Model file for the job. Use its own axes, mm. Give positions to 0.01 mm unless a question says otherwise; leave off trailing zeros. Write each loop counter-clockwise with the first axis right and the second up, starting at its lowest first coordinate (ties: lowest second). Pieces come first, ordered by that corner, then holes. Notation, with made-up numbers: (78.5, -13.75) - (109.5, -13.75) arc R14 cw to (109.5, -8.75) - close; hole circle Ø9 at (27.5, -10.75). An arc over 180 degrees is marked (long way). Use a Markdown table: item, result. Add a question column.
```python
from build123d import *

# Parameters (mm, degrees)
SKETCH_1_W          = 77.1
SKETCH_1_H          = 60
SKETCH_1_R          = 4.1
SKETCH_1_R_2        = 1.6
SKETCH_1_W_2        = 3.1
SKETCH_1_H_2        = 10
EXTRUDE_1_DEPTH     = 3
SKETCH_2_R          = 1.55
SKETCH_2_W          = 21.45
SKETCH_2_H          = 17
CUT_EXTRUDE_1_DEPTH = 49.939784429
SKETCH_3_R          = 4.1
EXTRUDE_2_DEPTH     = 3
FILLET_1_R          = 3


with BuildPart() as part:
    # 草图1 → 凸台-拉伸1 (new body)
    with BuildSketch(Plane.XY):
        Rectangle(SKETCH_1_W, SKETCH_1_H)
        Circle(SKETCH_1_R, mode=Mode.SUBTRACT)
        with Locations((34, 0)):
            Circle(SKETCH_1_R_2, mode=Mode.SUBTRACT)
        with Locations((-34, 0)):
            Circle(SKETCH_1_R_2, mode=Mode.SUBTRACT)
        with Locations((34, -20)):
            Rectangle(SKETCH_1_W_2, SKETCH_1_H_2, mode=Mode.SUBTRACT)
        with Locations((-34, 20)):
            Rectangle(SKETCH_1_W_2, SKETCH_1_H_2, mode=Mode.SUBTRACT)
        with Locations((-34, -20)):
            Rectangle(SKETCH_1_W_2, SKETCH_1_H_2, mode=Mode.SUBTRACT)
        with Locations((34, 20)):
            Rectangle(SKETCH_1_W_2, SKETCH_1_H_2, mode=Mode.SUBTRACT)
    extrude(amount=EXTRUDE_1_DEPTH)

    # 草图2 → 切除-拉伸1 (cut, through all)
    with BuildSketch(Plane.XY.offset(3)):
        with Locations((-34, 25)):
            Circle(SKETCH_2_R)
        with Locations((-34, 15)):
            Circle(SKETCH_2_R)
        with Locations((34, 25)):
            Circle(SKETCH_2_R)
        with Locations((34, 15)):
            Circle(SKETCH_2_R)
        with Locations((34, -15)):
            Circle(SKETCH_2_R)
        with Locations((34, -25)):
            Circle(SKETCH_2_R)
        with Locations((-34, -15)):
            Circle(SKETCH_2_R)
        with Locations((-34, -25)):
            Circle(SKETCH_2_R)
        with Locations((-15.725, 13.5)):
            Rectangle(SKETCH_2_W, SKETCH_2_H)
        with Locations((15.725, 13.5)):
            Rectangle(SKETCH_2_W, SKETCH_2_H)
        with Locations((-15.725, -13.5)):
            Rectangle(SKETCH_2_W, SKETCH_2_H)
        with Locations((15.725, -13.5)):
            Rectangle(SKETCH_2_W, SKETCH_2_H)
    extrude(amount=-CUT_EXTRUDE_1_DEPTH, mode=Mode.SUBTRACT)

    # 草图3 → 凸台-拉伸2 (add)
    # profile 1 of 2: a face of its own
    with BuildSketch(Plane.XY.offset(3)):
        Polygon((-38.55, 30), (-53.55, 12.123696111), (-53.55, -12.123696111), (-38.55, -30), align=None)
        with Locations((-46.5, 0)):
            Circle(SKETCH_3_R, mode=Mode.SUBTRACT)
        with BuildLine():
            Line((-40.55, 19.837873681), (-49.55, 9.112091347))
            Line((-49.55, 9.112091347), (-49.55, 7.503832354))
            ThreePointArc((-49.55, 7.503832354), (-44.736420639, 7.905680732), (-40.55, 5.496135006))
            Line((-40.55, 5.496135006), (-40.55, 19.837873681))
        make_face(mode=Mode.SUBTRACT)
        with BuildLine():
            Line((-49.55, -7.503832354), (-49.55, -9.112091347))
            Line((-49.55, -9.112091347), (-40.55, -19.837873681))
            Line((-40.55, -19.837873681), (-40.55, -5.496135006))
            ThreePointArc((-40.55, -5.496135006), (-44.736420639, -7.905680732), (-49.55, -7.503832354))
        make_face(mode=Mode.SUBTRACT)
    # profile 2 of 2: a face of its own
    with BuildSketch(Plane.XY.offset(3)):
        Polygon((53.55, -12.123696111), (38.55, -30), (38.55, 30), (53.55, 12.123696111), align=None)
        with Locations(Location((46.5, 0, 0), (0, 0, 180))):
            Circle(SKETCH_3_R, mode=Mode.SUBTRACT)
        with BuildLine():
            Line((40.55, -19.837873681), (40.55, -5.496135006))
            ThreePointArc((40.55, -5.496135006), (44.736420639, -7.905680732), (49.55, -7.503832354))
            Line((49.55, -7.503832354), (49.55, -9.112091347))
            Line((49.55, -9.112091347), (40.55, -19.837873681))
        make_face(mode=Mode.SUBTRACT)
        with BuildLine():
            Line((40.55, 19.837873681), (49.55, 9.112091347))
            Line((49.55, 9.112091347), (49.55, 7.503832354))
            ThreePointArc((49.55, 7.503832354), (44.736420639, 7.905680732), (40.55, 5.496135006))
            Line((40.55, 5.496135006), (40.55, 19.837873681))
        make_face(mode=Mode.SUBTRACT)
    extrude(amount=-EXTRUDE_2_DEPTH)

    # 圆角1
    fillet_1_edges = [part.edges().sort_by_distance(p)[0] for p in [
        (26.45, 5, 1.5),
        (5, 5, 1.5),
        (5, 22, 1.5),
        (26.45, 22, 1.5),
        (-26.45, -22, 1.5),
        (-26.45, -5, 1.5),
        (-5, -5, 1.5),
        (-5, -22, 1.5),
        (26.45, -22, 1.5),
        (5, -22, 1.5),
        (5, -5, 1.5),
        (26.45, -5, 1.5),
        (-26.45, 5, 1.5),
        (-26.45, 22, 1.5),
        (-5, 22, 1.5),
        (-5, 5, 1.5),
    ]]
    fillet(fillet_1_edges, radius=FILLET_1_R)


solid = part.part
```
(1) Probe probe 1 along X at (y, z) = (9, 2.4); probe 2 along Y at (x, z) = (34, 0.75); probe 3 along Y at (x, z) = (-17, 0.2). List the from-to ranges inside material, lowest first. Write a range as [from, to].
(2) Two-plate mould, pull along X, no slides. Class faces 1 (the flat face through (53.55, 0, 2)), 2 (the flat face through (-1, 30, 1)), 3 (the cylindrical face through (25.59, 21.1, 1.48)): +X half, -X half, draft (parallel to the pull), parting line (faces both ways), or undercut.
(3) Flat gauge pins, fed straight in: pin 1 (1.5 mm diameter, centred on y = 20.5, z = 2, fed in from -X); pin 2 (0.9 mm diameter, centred on y = 20, z = 1.5, fed in from -X); pin 3 (1.5 mm diameter, centred on y = -18, z = 2, fed in from +X); pin 4 (6.5 mm diameter, centred on x = 46.5, y = 0, fed in from -Z). Where does each tip first touch, or does it go through?
(4) Band-saw the part on C-C (x = 34). Write the cut outline in (y, z).
(5) Band-saw the part on D-D (x = 0). Write the cut outline in (y, z), then the cut area to 3 significant figures.
(6) Band-saw the part on B-B (y = 0). Write the cut outline in (x, z), then the cut area to 3 significant figures.
(7) Band-saw the part on A-A (x = -17). Write the cut outline in (y, z).
Model answer:
| question | item | result |
|---|---|---|
| 1 | probe 1 | x = [-53.55, -49.55], [-40.55, -26.45], [-5, 5], [26.45, 40.55], [49.55, 53.55] |
| 1 | probe 2 | y = [-30, -26.55], [-13.45, -1.6], [1.6, 13.45], [26.55, 30] |
| 1 | probe 3 | y = [-30, -22], [-5, 5], [22, 30] |
| 2 | face 1 | +X half |
| 2 | face 2 | draft |
| 2 | face 3 | undercut |
| 3 | pin 1 | stops at x = -47.15 |
| 3 | pin 2 | stops at x = -47.32 |
| 3 | pin 3 | stops at x = 49.25 |
| 3 | pin 4 | passes through |
| 4 | outline | (-30, 0) - (-26.55, 0) - (-26.55, 3) - (-30, 3) - close; (-13.45, 0) - (-1.6, 0) - (-1.6, 3) - (-13.45, 3) - close; (1.6, 0) - (13.45, 0) - (13.45, 3) - (1.6, 3) - close; (26.55, 0) - (30, 0) - (30, 3) - (26.55, 3) - close |
| 5 | outline | (-30, 0) - (-4.1, 0) - (-4.1, 3) - (-30, 3) - close; (4.1, 0) - (30, 0) - (30, 3) - (4.1, 3) - close |
| 5 | area | 155 mm^2 |
| 6 | outline | (-53.55, 0) - (-50.6, 0) - (-50.6, 3) - (-53.55, 3) - close; (-42.4, 0) - (-35.6, 0) - (-35.6, 3) - (-42.4, 3) - close; (-32.4, 0) - (-4.1, 0) - (-4.1, 3) - (-32.4, 3) - close; (4.1, 0) - (32.4, 0) - (32.4, 3) - (4.1, 3) - close; (35.6, 0) - (42.4, 0) - (42.4, 3) - (35.6, 3) - close; (50.6, 0) - (53.55, 0) - (53.55, 3) - (50.6, 3) - close |
| 6 | area | 228 mm^2 |
| 7 | outline | (-30, 0) - (-22, 0) - (-22, 3) - (-30, 3) - close; (-5, 0) - (5, 0) - (5, 3) - (-5, 3) - close; (22, 0) - (30, 0) - (30, 3) - (22, 3) - close |
